Read the model definition and answer for the solid it produces. Units are mm, in the model's axes. Face numbers are marked on the shaded views. Give positions to 0.01 mm unless a question says otherwise; leave off trailing zeros. Order: outer loops, then holes, each group sorted by start corner. A loop starts at its lowest first (then second) coordinate and runs counter-clockwise, first axis right, second up. Notation, with made-up numbers: (21.25, 39) - (76.25, 39) arc R23 cw to (76.25, 67) - close; hole circle Ø11 at (19, 61.5). An arc over 180 degrees is marked (long way). One line per item, written item: value. Start each with the question number.
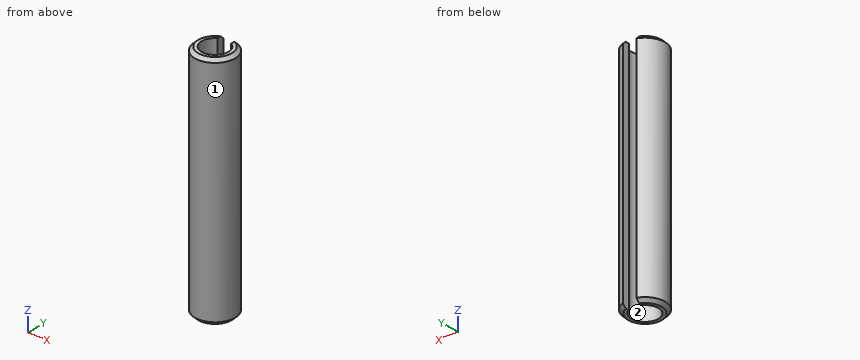
```python
from build123d import *

# Parameters (mm, degrees)
EXTRUSION2_DEPTH = 35
CHANFREIN1_SIZE  = 0.5


with BuildPart() as part:
    # Esquisse1 → Extrusion2 (new body)
    with BuildSketch(Plane.XY):
        with BuildLine():
            Line((-1, 2.828427125), (-1, 1.732050808))
            ThreePointArc((-1, 1.732050808), (0, -2), (1, 1.732050808))
            Line((1, 1.732050808), (1, 2.828427125))
            ThreePointArc((1, 2.828427125), (0, -3), (-1, 2.828427125))
        make_face()
    extrude(amount=EXTRUSION2_DEPTH)

    # Chanfrein1
    chanfrein1_edges = [part.edges().sort_by_distance(p)[0] for p in [
        (0, -3, 35),
        (0, -3, 0),
    ]]
    chamfer(chanfrein1_edges, length=CHANFREIN1_SIZE)


solid = part.part
```
1) The mould has two halves that part along X. Classify the marked faces 1 and 2: +X half, -X half, draft (parallel to the pull), parting line (faces both ways), or undercut.
2) Find the intervals of material crossed by probe 1 along X at (y, z) = (0.05, 13.5); probe 2 along Y at (x, z) = (0, 16); probe 3 along Y at (x, z) = (-1.5, 19.5), in increasing order. Write a range as from..to.
3) Section C-C on z = 5 is taken. Write down the section's boundary in (x, y), plus the area to 3 significant figures.
4) Section B-B on x = 0 is taken. Write down the section's boundary in (y, z).
5) Each of these flat-tipped pins is pushed along its axis until it touches: pin 1 (1 mm diameter, centred on x = 0, y = 1, fed in from +Z); pin 2 (1 mm diameter, centred on x = 1, z = 12.5, fed in from -Y); pin 3 (1 mm diameter, centred on y = 1.5, z = 23, fed in from +X); pin 4 (0.9 mm diameter, centred on y = 2, z = 10, fed in from -X). Where does it stop, or does it pass through?
6) Section A-A on y = 0 is taken. Write down the section's boundary in (x, z).
Solved:
1. face 1: parting line
1. face 2: undercut
2. probe 1: x = -3..-2, 2..3
2. probe 2: y = -3..-2
2. probe 3: y = -2.6..-1.32, 1.32..2.6
3. outline: (-1, 1.73) - (-1, 2.83) arc R3 ccw (long way) to (1, 2.83) - (1, 1.73) arc R2 cw (long way) to start
3. area: 13.6 mm2
4. outline: (-3, 0.5) - (-2.5, 0) - (-2, 0) - (-2, 35) - (-2.5, 35) - (-3, 34.5) - close
5. pin 1: passes through
5. pin 2: stops at y = -2.96
5. pin 3: stops at x = 2.83
5. pin 4: stops at x = -2.57
6. outline: (-3, 0.5) - (-2.5, 0) - (-2, 0) - (-2, 35) - (-2.5, 35) - (-3, 34.5) - close; (2, 0) - (2.5, 0) - (3, 0.5) - (3, 34.5) - (2.5, 35) - (2, 35) - close
